from build123d import *

# Parameters (mm, degrees)
F0_W     = 77
F0_H     = 65
F0_R     = 9.5
F0_R_2   = 3
F0_W_2   = 0.5
F1_DEPTH = 25
F2_R     = 3
F3_T     = 2.4
F4_DEPTH = 2.4
F5_W     = 2.4
F5_H     = 69.8
F6_DEPTH = 27.078461


with BuildPart() as f1:
    # F0 (on Top) → F1 (new body)
    with BuildSketch(Plane.XY):
        with Locations((-42.871317, 11.163915)):
            Rectangle(F0_W, F0_H)
        with Locations((-65.871317, -6.405085)):
            Circle(F0_R, mode=Mode.SUBTRACT)
        with Locations((-44.871317, -6.405085)):
            Circle(F0_R, mode=Mode.SUBTRACT)
        with Locations((-29.871317, -6.405085)):
            Circle(F0_R_2, mode=Mode.SUBTRACT)
        with Locations((-14.871317, -6.405085)):
            Circle(F0_R, mode=Mode.SUBTRACT)
        with Locations((-65.871317, -6.405085)):
            Circle(F0_R)
        with Locations((-44.871317, -6.405085)):
            Circle(F0_R)
        with Locations((-29.871317, -6.405085)):
            Circle(F0_R_2)
        with Locations((-14.871317, -6.405085)):
            Circle(F0_R)
        with Locations((-4.121317, 11.163915)):
            Rectangle(F0_W_2, F0_H)
    extrude(amount=F1_DEPTH)

    # F2
    f2_edges = [f1.edges().sort_by_distance(p)[0] for p in [
        (-81.371317, -21.336085, 12.5),
        (-81.371317, 43.663915, 12.5),
        (-42.621317, 43.663915, 0),
        (-81.371317, 11.163915, 0),
        (-42.621317, -21.336085, 0),
    ]]
    fillet(f2_edges, radius=F2_R)

    # F3
    f3_openings = [f1.faces().sort_by_distance(p)[0] for p in [
        (-42.592095, 11.163915, 25),
    ]]
    offset(amount=F3_T, openings=f3_openings)

    # F0 (on Top) → F4 (cut, through all)
    with BuildSketch(Plane.XY):
        with Locations((-14.871317, -6.405085)):
            Circle(F0_R)
        with Locations((-29.871317, -6.405085)):
            Circle(F0_R_2)
        with Locations((-44.871317, -6.405085)):
            Circle(F0_R)
        with Locations((-65.871317, -6.405085)):
            Circle(F0_R)
    extrude(amount=-F4_DEPTH, mode=Mode.SUBTRACT)

    # F5 (on face) → F6 (cut, through all)
    with BuildSketch(Plane.XY.offset(25)):
        with Locations((-2.671317, 11.163915)):
            Rectangle(F5_W, F5_H)
    extrude(amount=-F6_DEPTH, mode=Mode.SUBTRACT)

    # F7: F1 across face


with BuildPart() as f1_1:
    add(f1.part)
    add(f1.part.mirror(Plane(origin=(-3.871317, 11.163915, 5.251674), x_dir=(0, 1, 0), z_dir=(1, 0, 0))))


solid = f1_1.part
Model file for the job. Use its own axes, mm. A direction names the side the tool comes from. Round coordinates to 2 decimals unless told otherwise and drop trailing zeros. Loops run counter-clockwise (first coordinate to the right, second up) from the corner with the lowest first, then second, coordinate; pieces in that order, holes last. Notation, with made-up numbers: (34.25, -8) -> (67.25, -8) arc R38 cw to (67.25, 30) -> close; hole circle Ø7 at (61.25, 88.5). An arc over 180 degrees is marked (long way). Answer as CSV lines item,"result". Start each with the question number.
1) Slice it at C-C (x = -68.5). List the corners of the cut face in (y, z), plus the area to 3 significant figures.
2) Slice it at B-B (y = 31). List the corners of the cut face in (x, z), plus the area to 3 significant figures.
3) Probe line 1 along X through (y, z) = (-0.5, 21.5); line 2 along Y through (x, z) = (-29, 16.5); line 3 along Z through (x, y) = (0.5, -16.5). List the from-to ranges inside material, lowest first.
4) Tool access for faces 4 (the face through (-54.362, -5.987, -1.183)), 5 (the face through (-80.52, -20.43, 14.15)): list every direction of +Z, -Z, +X, -X, +Y, -Y with a clear straight run to the whole face (end or side of a thin tool).
5) Mould opens along X. For faces 1 (the face through (-5, 43.664, 14)), 2 (the face through (-4.914, -22.196, -0.776)), 3 (the face through (76.029, 11, 14)) say: +X half, -X half, draft (parallel to the pull), parting line (faces both ways), or undercut.
6) Pin check, flat tips, straight feed: P1, Ø15, axis at x = -65.87, y = -6.41, coming from the +Z side; P2, Ø17.5, axis at x = 18.5, y = 10.5, coming from the +Z side. Stop position of each tip, or through.
7) Slice it at A-A (z = 20.5). List the corners of the cut face in (x, y).
8) Slice it at D-D (x = 4). List the corners of the cut face in (y, z), plus the area to 3 significant figures.
Filled in:
1,outline,"(-23.74, 3) arc R5.4 ccw to (-18.34, -2.4) -> (-15.53, -2.4) -> (-15.53, 0) -> (-18.34, 0) arc R3 cw to (-21.34, 3) -> (-21.34, 25) -> (-23.74, 25) -> close; (2.72, -2.4) -> (40.66, -2.4) arc R5.4 ccw to (46.06, 3) -> (46.06, 25) -> (43.66, 25) -> (43.66, 3) arc R3 cw to (40.66, 0) -> (2.72, 0) -> close"
1,area,"235 mm2"
2,outline,"(-83.77, 3) arc R5.4 ccw to (-78.37, -2.4) -> (70.63, -2.4) arc R5.4 ccw to (76.03, 3) -> (76.03, 25) -> (73.63, 25) -> (73.63, 3) arc R3 cw to (70.63, 0) -> (-78.37, 0) arc R3 cw to (-81.37, 3) -> (-81.37, 25) -> (-83.77, 25) -> close"
2,area,"495 mm2"
3,line 1,"x = -83.77 to -81.37, 73.63 to 76.03"
3,line 2,"y = -23.74 to -21.34, 43.66 to 46.06"
3,line 3,"z = -2.4 to 0"
4,face 4,"+Z, -Z"
4,face 5,"+Z"
5,face 1,"undercut"
5,face 2,"draft"
5,face 3,"+X half"
6,P1,"passes through"
6,P2,"stops at z = 0"
7,outline,"(-83.77, -18.34) arc R5.4 ccw to (-78.37, -23.74) -> (70.63, -23.74) arc R5.4 ccw to (76.03, -18.34) -> (76.03, 40.66) arc R5.4 ccw to (70.63, 46.06) -> (-78.37, 46.06) arc R5.4 ccw to (-83.77, 40.66) -> close; hole (-81.37, -18.34) arc R3 ccw to (-78.37, -21.34) -> (70.63, -21.34) arc R3 ccw to (73.63, -18.34) -> (73.63, 40.66) arc R3 ccw to (70.63, 43.66) -> (-78.37, 43.66) arc R3 ccw to (-81.37, 40.66) -> close"
8,outline,"(-23.74, 3) arc R5.4 ccw to (-18.34, -2.4) -> (-15.38, -2.4) -> (-15.38, 0) -> (-18.34, 0) arc R3 cw to (-21.34, 3) -> (-21.34, 25) -> (-23.74, 25) -> close; (2.56, -2.4) -> (40.66, -2.4) arc R5.4 ccw to (46.06, 3) -> (46.06, 25) -> (43.66, 25) -> (43.66, 3) arc R3 cw to (40.66, 0) -> (2.56, 0) -> close"
8,area,"236 mm2"
